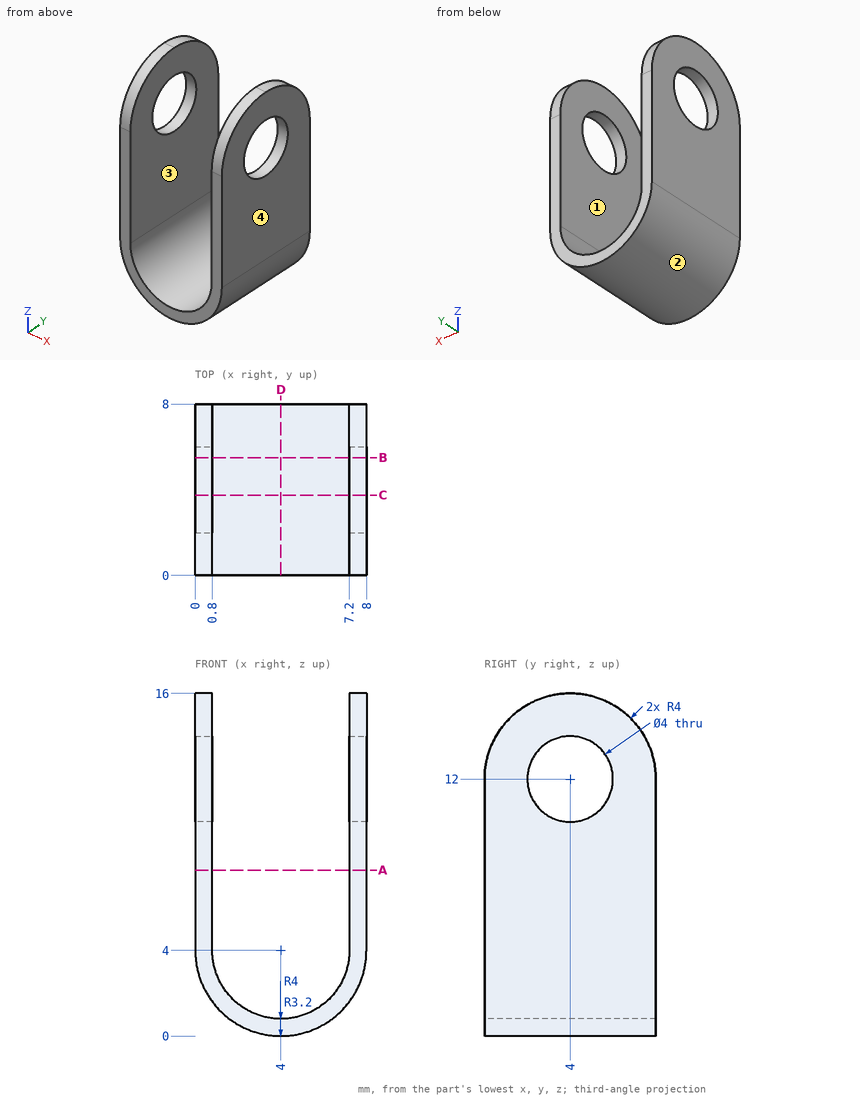
Source: three-view drawing plus pictorial views. Frame: mm from the lowest corner of the part. Give positions to 0.01 mm unless a question says otherwise; leave off trailing zeros. Order: outer loops, then holes, each group sorted by start corner. A loop starts at its lowest first (then second) coordinate and runs counter-clockwise, first axis right, second up. Notation, with made-up numbers: M -15.75,-11 L 1.25,-11 A19 ccw 1.25,3 Z; hole C 74.5,17 d10. An arc over 180 degrees is marked long. Return JSON: item names as keys, results as strings.
1) Mould query, pull axis X, two halves, no side actions, for the marked faces 1, 2, 3 and 4. Classes: released by +X, released by -X, zero draft, split by the parting line, or undercut.
Taken from the geometry:
{"face 1": "undercut", "face 2": "split by the parting line", "face 3": "undercut", "face 4": "released by +X"}
2) Contact query for flat-ended pins moving along their axis: pin 1 (3 mm diameter, centred on x = 7, y = 2.5, fed in from -Z); pin 2 (4 mm diameter, centred on x = 1.5, y = 1.5, fed in from -Z); pin 3 (1.5 mm diameter, centred on y = 5.5, z = 2.5, fed in from +X). Output: stop coordinate, or through.
Taken from the geometry:
{"pin 1": "stops at z = 0.29", "pin 2": "stops at z = 0.03", "pin 3": "stops at x = 7.93"}
3) Section query B-B on y = 5.5. Output: boundary loops of the cut face in (x, z).
Taken from the geometry:
{"outline": "M 0,4 A4 ccw 8,4 L 8,10.68 L 7.2,10.68 L 7.2,4 A3.2 cw 0.8,4 L 0.8,10.68 L 0,10.68 Z; M 0,13.32 L 0.8,13.32 L 0.8,15.71 L 0,15.71 Z; M 7.2,13.32 L 8,13.32 L 8,15.71 L 7.2,15.71 Z"}
4) Section query D-D on x = 4. Output: boundary loops of the cut face in (y, z).
Taken from the geometry:
{"outline": "M 0,0 L 8,0 L 8,0.8 L 0,0.8 Z"}
5) Section query C-C on y = 3.75. Output: boundary loops of the cut face in (x, z).
Taken from the geometry:
{"outline": "M 0,4 A4 ccw 8,4 L 8,10.02 L 7.2,10.02 L 7.2,4 A3.2 cw 0.8,4 L 0.8,10.02 L 0,10.02 Z; M 0,13.98 L 0.8,13.98 L 0.8,15.99 L 0,15.99 Z; M 7.2,13.98 L 8,13.98 L 8,15.99 L 7.2,15.99 Z"}
6) Section query A-A on z = 7.75. Output: boundary loops of the cut face in (x, y).
Taken from the geometry:
{"outline": "M 0,0 L 0.8,0 L 0.8,8 L 0,8 Z; M 7.2,0 L 8,0 L 8,8 L 7.2,8 Z"}
7) Line query: L1, parallel to X at y = 7.75, z = 6.75; L2, parallel to Y at x = 0.35, z = 12; L3, parallel to X at y = 1, z = 1.25 (1 decimal). Output: solid intervals per line, ascending. Write a range as [from, to].
Taken from the geometry:
{"L1": "x = [0, 0.8], [7.2, 8]", "L2": "y = [0, 2], [6, 8]", "L3": "x = [1.1, 2.4], [5.6, 6.9]"}
